Check sheet for the drawn part. Datum: minimum x, y, z corner. Units: mm. A direction names the side the tool comes from. Round coordinates to 2 decimals unless told otherwise and drop trailing zeros. Order: outer loops, then holes, each group sorted by start corner. A loop starts at its lowest first (then second) coordinate and runs counter-clockwise, first axis right, second up. Notation, with made-up numbers: (81, 77) -> (126, 77) arc R23 cw to (126, 97) -> close; hole circle Ø4 at (35.5, -15.5). An arc over 180 degrees is marked (long way). Answer in a Markdown table with one row per item.
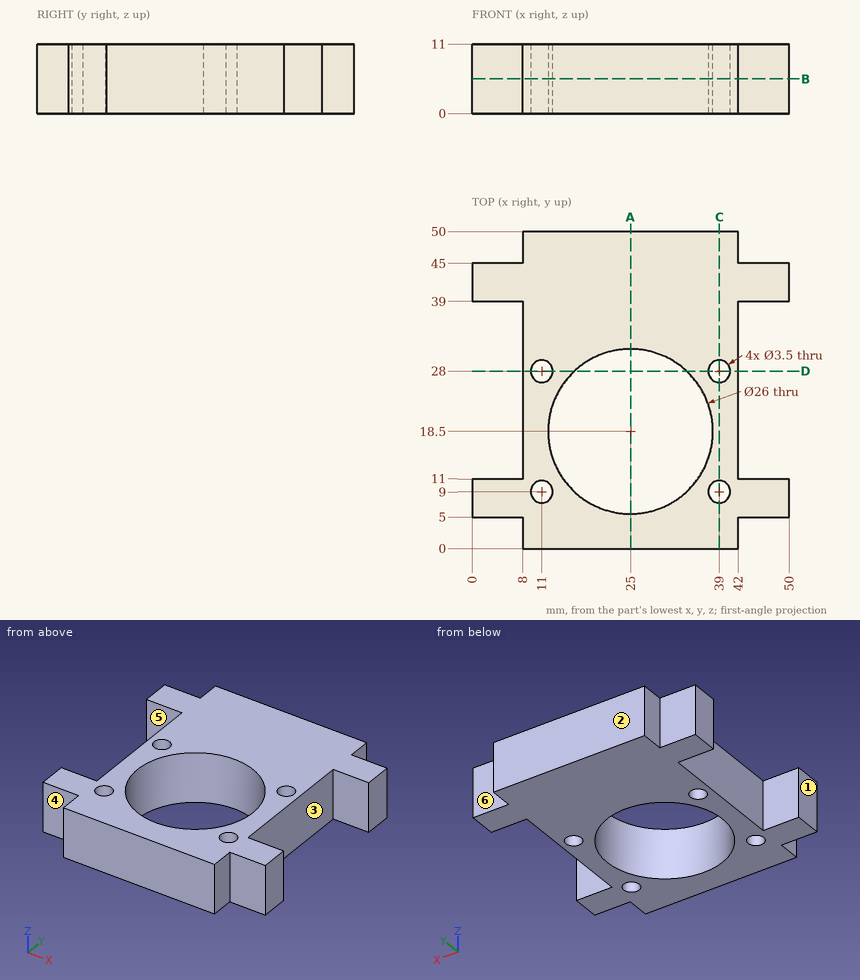
(1) Section check D-D on y = 28. Record the boundary of the cut face in (x, z), plus the area to 3 significant figures.
Solutions:
| item | result |
|---|---|
| outline | (8, 0) -> (9.25, 0) -> (9.25, 11) -> (8, 11) -> close; (12.75, 0) -> (16.13, 0) -> (16.13, 11) -> (12.75, 11) -> close; (33.87, 0) -> (37.25, 0) -> (37.25, 11) -> (33.87, 11) -> close; (40.75, 0) -> (42, 0) -> (42, 11) -> (40.75, 11) -> close |
| area | 102 mm^2 |
(2) Tool access check on the marked faces 4, 5 and 6. Record the directions out of +Z, -Z, +X, -X, +Y, -Y that give a thin tool (end or side, any length) a straight path to the whole face; none if there is none.
Solutions:
| item | result |
|---|---|
| face 4 | +Z, -Z, -X, -Y |
| face 5 | +Z, -Z, -X |
| face 6 | +Z, -Z, +X, +Y |
(3) Section check B-B on z = 5.5. Record the boundary of the cut face in (x, y).
Solutions:
| item | result |
|---|---|
| outline | (0, 5) -> (8, 5) -> (8, 0) -> (42, 0) -> (42, 5) -> (50, 5) -> (50, 11) -> (42, 11) -> (42, 39) -> (50, 39) -> (50, 45) -> (42, 45) -> (42, 50) -> (8, 50) -> (8, 45) -> (0, 45) -> (0, 39) -> (8, 39) -> (8, 11) -> (0, 11) -> close; hole circle Ø3.5 at (11, 9); hole circle Ø3.5 at (11, 28); hole circle Ø26 at (25, 18.5); hole circle Ø3.5 at (39, 9); hole circle Ø3.5 at (39, 28) |
(4) Depth check by flat-ended pin: pin 1 Ø1.5 at (y, z) = (2.5, 7) entering from -X; pin 2 Ø3 at (y, z) = (35, 7) entering from +X; pin 3 Ø3 at (x, y) = (11, 9) entering from -Z (1 decimal); pin 4 Ø2.5 at (x, z) = (46.5, 4) entering from +Y. Enter the tip coordinate at first touch or a pass-through.
Solutions:
| item | result |
|---|---|
| pin 1 | x = 8 |
| pin 2 | x = 42 |
| pin 3 | through |
| pin 4 | y = 45 |
(5) Section check A-A on x = 25. Record the boundary of the cut face in (y, z), plus the area to 3 significant figures.
Solutions:
| item | result |
|---|---|
| outline | (0, 0) -> (5.5, 0) -> (5.5, 11) -> (0, 11) -> close; (31.5, 0) -> (50, 0) -> (50, 11) -> (31.5, 11) -> close |
| area | 264 mm^2 |
(6) Section check C-C on x = 39. Record the boundary of the cut face in (y, z).
Solutions:
| item | result |
|---|---|
| outline | (0, 0) -> (7.25, 0) -> (7.25, 11) -> (0, 11) -> close; (10.75, 0) -> (26.25, 0) -> (26.25, 11) -> (10.75, 11) -> close; (29.75, 0) -> (50, 0) -> (50, 11) -> (29.75, 11) -> close |
(7) Scan lines: probe 1 along Y at (x, z) = (39, 4); probe 2 along Y at (x, z) = (25, 8.25); probe 3 along Y at (x, z) = (7, 3.25). Record each from-to range of solid material in increasing order. Write a range as from..to.
Solutions:
| item | result |
|---|---|
| probe 1 | 0..7.25, 10.75..26.25, 29.75..50 |
| probe 2 | 0..5.5, 31.5..50 |
| probe 3 | 5..11, 39..45 |
(8) Draft check along Y on the marked faces 1, 2 and 3. Enter one of: pulls with the +Y half, pulls with the -Y half, needs draft (parallel to the pull), parting line crosses it, or undercut.
Solutions:
| item | result |
|---|---|
| face 1 | needs draft |
| face 2 | pulls with the +Y half |
| face 3 | undercut |
